Build history of the part. All positions in model axes, mm. Face numbers are marked on the shaded views. Give positions to 0.01 mm unless a question says otherwise; leave off trailing zeros. Write each question's results on one line, items separated by ' | '. Start each with the question number.
from build123d import *

# Parameters (mm, degrees)
SKETCH1_W           = 59
SKETCH1_H           = 49.5
SKETCH1_R           = 3
BOSS_EXTRUDE1_DEPTH = 1.5
BOSS_EXTRUDE2_DEPTH = 49.5
CUT_EXTRUDE1_DEPTH  = 1
CUT_EXTRUDE3_DEPTH  = 65.105869466
BOSS_EXTRUDE3_START = 0.5
SKETCH5_R           = 3
BOSS_EXTRUDE3_DEPTH = 0.5
SKETCH6_W           = 3.5
SKETCH6_H           = 2.563301414
CUT_EXTRUDE4_DEPTH  = 0.5
CHAMFER3_SIZE       = 1.5


with BuildPart() as part:
    # Sketch1 → Boss-Extrude1 (new body)
    with BuildSketch(Plane(origin=(0, 0, 0), x_dir=(1, 0, 0), z_dir=(0, 1, 0))):
        Rectangle(SKETCH1_W, SKETCH1_H)
        with Locations(Location((0, 0, 0), (0, 0, 270))):
            Circle(SKETCH1_R, mode=Mode.SUBTRACT)
    extrude(amount=BOSS_EXTRUDE1_DEPTH)

    # Sketch2 → Boss-Extrude2 (add)
    with BuildSketch(Plane(origin=(0, 0, -24.75), x_dir=(-1, 0, 0), z_dir=(0, 0, -1))):
        Polygon((-29.5, 1.5), (29.5, 1.5), (29.5, 2.5), (28.32, 4), (27.14, 2.5), (25.96, 4), (24.78, 2.5), (23.6, 4), (22.42, 2.5), (21.24, 4), (20.06, 2.5), (18.88, 4), (17.7, 2.5), (16.52, 4), (15.34, 2.5), (14.16, 4), (12.98, 2.5), (11.8, 4), (10.62, 2.5), (9.44, 4), (8.26, 2.5), (7.08, 4), (5.9, 2.5), (4.72, 4), (3.54, 2.5), (2.36, 4), (1.18, 2.5), (0, 4), (-1.18, 2.5), (-2.36, 4), (-3.54, 2.5), (-4.72, 4), (-5.9, 2.5), (-7.08, 4), (-8.26, 2.5), (-9.44, 4), (-10.62, 2.5), (-11.8, 4), (-12.98, 2.5), (-14.16, 4), (-15.34, 2.5), (-16.52, 4), (-17.7, 2.5), (-18.88, 4), (-20.06, 2.5), (-21.24, 4), (-22.42, 2.5), (-23.6, 4), (-24.78, 2.5), (-25.96, 4), (-27.14, 2.5), (-28.32, 4), (-29.5, 2.5), align=None)
    extrude(amount=-BOSS_EXTRUDE2_DEPTH)

    # Sketch3 → Cut-Extrude1 (cut)
    with BuildSketch(Plane(origin=(0, 0, 0), x_dir=(-1, 0, 0), z_dir=(0, -1, 0))):
        with BuildLine():
            Line((-1.75, -2.436698586), (-1.75, -5))
            Line((-1.75, -5), (1.75, -5))
            Line((1.75, -5), (1.75, -2.436698586))
            ThreePointArc((1.75, -2.436698586), (0, 3), (-1.75, -2.436698586))
        make_face()
    extrude(amount=-CUT_EXTRUDE1_DEPTH, mode=Mode.SUBTRACT)

    # Sketch4 → Cut-Extrude3 (cut, through all)
    with BuildSketch(Plane(origin=(29.5, 0, 0), x_dir=(0, 0, -1), z_dir=(1, 0, 0))):
        with BuildLine():
            Line((-24, 4), (-24.75, 4))
            Line((-24.75, 4), (-24.75, 3.25))
            ThreePointArc((-24.75, 3.25), (-24.530330086, 3.780330086), (-24, 4))
        make_face()
    cut_extrude3 = extrude(amount=-CUT_EXTRUDE3_DEPTH, mode=Mode.SUBTRACT)

    # Mirror1: Cut-Extrude3 across plane
    add(cut_extrude3.mirror(Plane.XY), mode=Mode.SUBTRACT)

    # Sketch5 → Boss-Extrude3 (add)
    with BuildSketch(Plane.XZ.offset(-1.5).offset(BOSS_EXTRUDE3_START)):
        Circle(SKETCH5_R)
    extrude(amount=-BOSS_EXTRUDE3_DEPTH)

    # Sketch6 → Cut-Extrude4 (cut)
    with BuildSketch(Plane.XZ.offset(-1)):
        with Locations((0, 3.718349293)):
            Rectangle(SKETCH6_W, SKETCH6_H)
    extrude(amount=-CUT_EXTRUDE4_DEPTH, mode=Mode.SUBTRACT)

    # Chamfer3
    chamfer3_edges = [part.edges().sort_by_distance(p)[0] for p in [
        (0, 0, 5),
    ]]
    chamfer(chamfer3_edges, length=CHAMFER3_SIZE - 0.0001)  # a hair under: the kernel refuses the full size


solid = part.part
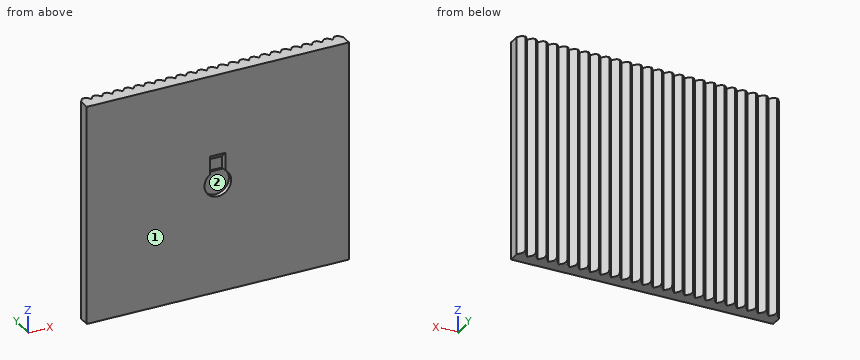
Item 1: Flat gauge pins, fed straight in: pin 1 Ø3.5 at (x, z) = (0, 0) entering from -Y; pin 2 Ø8 at (x, z) = (-9, 12) entering from +Y. Where does each tip first touch, or does it go through?
Item 2: Two-plate mould, pull along Z, no slides. Class the marked faces 1 and 2: +Z half, -Z half, draft (parallel to the pull), parting line (faces both ways), or undercut.
Item 3: Probe line 1 along X through (y, z) = (0.7, 0); line 2 along Z through (x, y) = (0, 0.25); line 3 along Y through (x, z) = (-2, -18). List the from-to ranges inside material, lowest first. Write a range as from..to.
Values found:
1) pin 1: stops at y = 1 | pin 2: stops at y = 4
2) face 1: draft | face 2: undercut
3) line 1: x = -29.5..-3, 3..29.5 | line 2: z = -24.75..-3, 6.25..24.75 | line 3: y = 0..3.54
